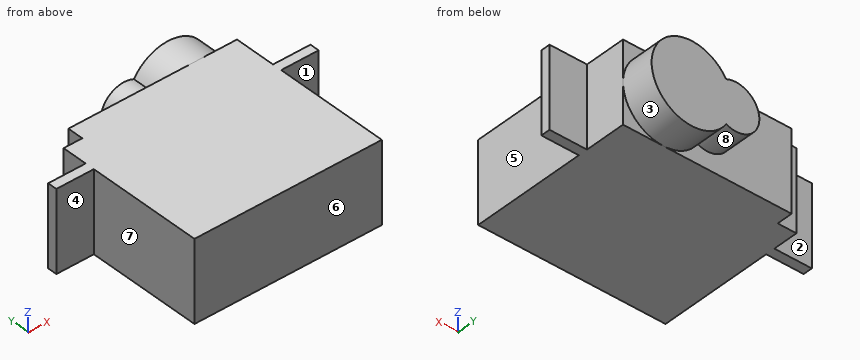
Autodesk Inventor part; units mm, degrees
ref_plane "YZ Plane" through (0, 0, 0) normal (1, 0, 0) x (0, 1, 0)
ref_plane "XZ Plane" through (0, 0, 0) normal (0, 1, 0) x (-1, 0, 0)
ref_plane "XY Plane" through (0, 0, 0) normal (0, 0, 1) x (1, 0, 0)
sketch "Sketch1" plane through (0, 0, 0) normal (0, 0, 1) x (1, 0, 0)
  line L0 (0, 0) -> (-20, 0)
  line L1 (-18, 17.7) -> (0, 17.7)
  line L2 (-20, 17.7) -> (-18, 17.7)
  line L3 (-18, 17.7) -> (-18, 16)
  line L4 (-18, 16) -> (-20, 16)
  line L5 (-20, 16) -> (-20, 13.3)
  line L6 (-20, 13.3) -> (-24, 13.3)
  line L7 (-24, 13.3) -> (-24, 12.3)
  line L8 (-24, 12.3) -> (-20, 12.3)
  line L9 (-20, 0) -> (-20, 12.3)
  line L10 (-20, 13.3) -> (-20, 16)
  line L11 (0, 13.3) -> (4, 13.3)
  line L12 (4, 13.3) -> (4, 12.3)
  line L13 (4, 12.3) -> (0, 12.3)
  line L14 (0, 0) -> (0, 12.3)
  line L15 (0, 13.3) -> (0, 17.7)
  dimension "d0" = 20
  dimension "d1" = 17.7
  dimension "d2" = 2
  dimension "d3" = 1.7
  dimension "d4" = 2.7
  dimension "d5" = 4
  dimension "d6" = 1
extrude "Extrusion1" add sketch "Sketch1" along normal blind 8.6
sketch "Sketch2" plane through (-18, 17.7, 0) normal (0, 1, 0) x (1, 0, 0)
  line L0 (18, 0) -> (0, 0)
  line L1 (0, 0) -> (0, -8.6)
  line L2 (18, -8.6) -> (0, -8.6)
  line L3 (18, 0) -> (18, -8.6)
  circle A0 centre (13.7, -4.3) radius 4.3
extrude "Extrusion2" add sketch "Sketch2" along normal blind 3.5 contours A0
sketch "Sketch3" plane through (-18, 17.7, 8.6) normal (0, 1, 0) x (1, 0, 0)
  line L0 (18, 8.6) -> (18, 4.3)
  line L1 (9, 8.6) -> (9, 0)
  line L2 (13.7, 8.6) -> (0, 8.6)
  line L3 (13.7, 0) -> (0, 0)
  line L4 (6.1752, 8.6) -> (10.4672, 8.6)
  line L5 (6.1752, 0) -> (10.4672, 0)
  circle A0 centre (9, 4.3) radius 2.5
  dimension "d11" = 9
  dimension "d12" = 5
extrude "Extrusion3" add sketch "Sketch3" along normal up to surface (3.5 mm away)
sketch "Sketch4" plane through (0, 0, 8.6) normal (0, 0, 1) x (1, 0, 0)
  line L0 (-24, 13.3) -> (-24, 12.3)
  line L1 (-20, 13.3) -> (-24, 13.3)
  line L2 (-20, 16) -> (-20, 13.3)
  line L3 (-18, 16) -> (-20, 16)
  line L4 (-18, 17.7) -> (-18, 16)
  line L5 (-4.3, 17.7) -> (-18, 17.7)
  line L6 (0, 17.7) -> (-4.3, 17.7)
  line L7 (0, 13.3) -> (0, 17.7)
  line L8 (4, 13.3) -> (0, 13.3)
  line L9 (4, 12.3) -> (4, 13.3)
  line L10 (0, 12.3) -> (4, 12.3)
  line L11 (0, 0) -> (0, 12.3)
  line L12 (-20, 0) -> (0, 0)
  line L13 (-20, 12.3) -> (-20, 0)
  line L14 (-24, 12.3) -> (-20, 12.3)
sketch "Sketch5" plane through (0, 0, 0) normal (1, 0, 0) x (0, 0, -1)
  line L0 (0, 0) -> (0, 12.3)
  line L1 (0, 12.3) -> (-8.6, 12.3)
  line L2 (-8.6, 0) -> (-8.6, 12.3)
  line L3 (0, 0) -> (-8.6, 0)
properties part number "Servo"
For this review, take the finished solid that the model builds, in its own axes (mm). Face numbers are marked on the shaded views. A direction names the side the tool comes from. Round coordinates to 2 decimals unless told otherwise and drop trailing zeros. Loops run counter-clockwise (first coordinate to the right, second up) from the corner with the lowest first, then second, coordinate; pieces in that order, holes last.
Q1. Add section D-D on x = -21.25. Write out the cut boundary in (y, z), plus the area to 3 significant figures.
Result sheet:
outline: (12.3, 0) - (13.3, 0) - (13.3, 8.6) - (12.3, 8.6) - close
area: 8.60 mm2
Q2. To check wall thickness, follow line 1 along Y through (x, z) = (-19.75, 1.25); line 2 along X through (y, z) = (3.75, 2); line 3 along Y through (x, z) = (-12, 4.25). State the ranges of each line that lie inside material, in increasing order.
Result sheet:
line 1: y = 0 to 16
line 2: x = -20 to 0
line 3: y = 0 to 17.7
Q3. Add section C-C on y = 14. Write out the cut boundary in (x, z).
Result sheet:
outline: (-20, 0) - (0, 0) - (0, 8.6) - (-20, 8.6) - close
Q4. Add section B-B on z = 6. Write out the cut boundary in (x, y).
Result sheet:
outline: (-24, 12.3) - (-20, 12.3) - (-20, 0) - (0, 0) - (0, 12.3) - (4, 12.3) - (4, 13.3) - (0, 13.3) - (0, 17.7) - (-0.35, 17.7) - (-0.35, 21.2) - (-10.83, 21.2) - (-10.83, 17.7) - (-18, 17.7) - (-18, 16) - (-20, 16) - (-20, 13.3) - (-24, 13.3) - close
Q5. Add section A-A on x = -11. Write out the cut boundary in (y, z).
Result sheet:
outline: (0, 0) - (17.7, 0) - (17.7, 2.8) - (21.2, 2.8) - (21.2, 5.8) - (17.7, 5.8) - (17.7, 8.6) - (0, 8.6) - close
Q6. Mouldability with a two-part tool opening along X and no side actions: class the marked faces 5, 6, 7 and 8 as +X half, -X half, draft (parallel to the pull), parting line (faces both ways), or undercut.
Result sheet:
face 5: +X half
face 6: draft
face 7: -X half
face 8: undercut
Q7. Insertion check: pin 1 Ø2 at (x, z) = (-16.5, 6) entering from +Y; pin 2 Ø3 at (x, z) = (2, 3.5) entering from -Y; pin 3 Ø1.2 at (x, z) = (1.5, 3.5) entering from +Y; pin 4 Ø6 at (x, y) = (-9.5, 18) entering from -Z. Each pin has a flat end and moves straight along its axis. Give the tip position at first contact, or say it passes through.
Result sheet:
pin 1: stops at y = 17.7
pin 2: stops at y = 12.3
pin 3: stops at y = 13.3
pin 4: stops at z = 0
Q8. Machinability: for the marked faces 1, 2, 3 and 4, which of the approach directions +Z, -Z, +X, -X, +Y, -Y give a long, thin tool a straight path to every point of the face, cutting with its end or side? Answer none if there is none.
Result sheet:
face 1: +Z, -Z, +X, -Y
face 2: +Z, -Z, -X, +Y
face 3: +Y
face 4: +Z, -Z, -X, -Y
